Check sheet for the modelled part. Datum: model origin and axes. Units: mm. Round coordinates to 2 decimals unless told otherwise and drop trailing zeros. Loops run counter-clockwise (first coordinate to the right, second up) from the corner with the lowest first, then second, coordinate; pieces in that order, holes last. Notation, with made-up numbers: (35, -2) -> (65, -2) arc R18 cw to (65, 19) -> close; hole circle Ø10 at (72, 4.25). An arc over 180 degrees is marked (long way). One line per item, written item: value. Start each with the question number.
1. Go/stop test with flat-tipped pins: pin 1 (0.7 mm diameter, centred on x = 0.5, y = -6, fed in from +Z); pin 2 (1.5 mm diameter, centred on x = 1.5, y = -3, fed in from -Z). Record where each tip stops, or that it passes through.
2. Cross-section at A-A on x = 0. Record the cut outline in (y, z), then the cut area to 3 significant figures.
3. Cross-section at B-B on z = 0.6. Record the cut outline in (x, y), then the cut area to 3 significant figures.
4. Material ranges on L1, parallel to Y at x = 0, z = 0.45; L2, parallel to Z at x = 1, y = -6.25; L3, parallel to Y at x = -2, z = 2.35, recorded low to high.
from build123d import *

# Parameters (mm, degrees)
SKETCH1_R           = 5
BOSS_EXTRUDE1_DEPTH = 2.7
BOSS_EXTRUDE2_DEPTH = 0.15
FILLET2_R           = 0.2


with BuildPart() as part:
    # Sketch1 → Boss-Extrude1 (new body)
    with BuildSketch(Plane.XY):
        with Locations(Location((0, 0, 0), (0, 0, 180))):
            Circle(SKETCH1_R)
    extrude(amount=BOSS_EXTRUDE1_DEPTH)

    # Sketch3 → Boss-Extrude2 (add)
    with BuildSketch(Plane(origin=(0, 0, 0), x_dir=(-1, 0, 0), z_dir=(0, 0, -1))):
        Polygon((1.25, -4.841229183), (1.25, -7.091229183), (-1.25, -7.091229183), (-1.25, -4.841229183), (-1.25, -4.179733262), (1.25, -4.179733262), align=None)
    extrude(amount=-BOSS_EXTRUDE2_DEPTH)

    # Fillet2
    fillet2_edges = [part.edges().sort_by_distance(p)[0] for p in [
        (5, 0, 2.7),
    ]]
    fillet(fillet2_edges, radius=FILLET2_R)


solid = part.part
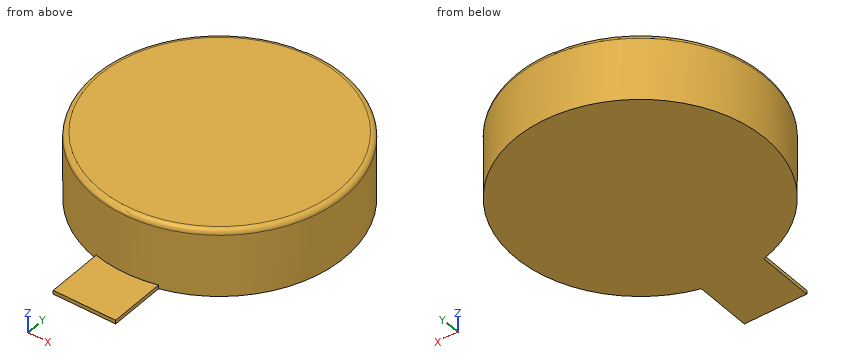
Taken from the geometry:
1. pin 1: stops at z = 0.15
1. pin 2: stops at z = 0
2. outline: (-7.09, 0) -> (5, 0) -> (5, 2.5) arc R0.2 ccw to (4.8, 2.7) -> (-4.8, 2.7) arc R0.2 ccw to (-5, 2.5) -> (-5, 0.15) -> (-7.09, 0.15) -> close
2. area: 27.3 mm2
3. outline: circle Ø10 at (0, 0)
3. area: 78.5 mm2
4. L1: y = -5 to 5
4. L2: z = 0 to 0.15
4. L3: y = -4.58 to 4.58
